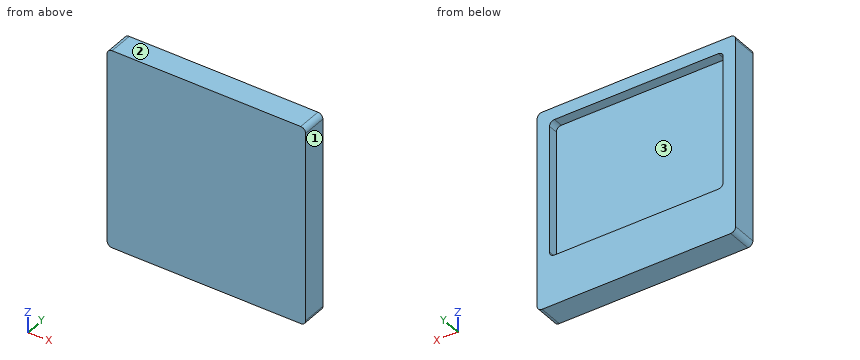
Autodesk Inventor part; units mm, degrees
ref_plane "YZ Plane" through (0, 0, 0) normal (1, 0, 0) x (0, 1, 0)
ref_plane "XZ Plane" through (0, 0, 0) normal (0, 1, 0) x (-1, 0, 0)
ref_plane "XY Plane" through (0, 0, 0) normal (0, 0, 1) x (1, 0, 0)
sketch "Sketch1" plane through (0, 0, 0) normal (0, 1, 0) x (-1, 0, 0)
  line L0 (0, 0) -> (80, 0)
  line L1 (80, 0) -> (80, -80)
  line L2 (80, -80) -> (0, -80)
  line L3 (0, -80) -> (0, 0)
  dimension "d0" = 80
  dimension "d1" = 80
extrude "Extrusion1" add sketch "Sketch1" along normal blind 6
sketch "Sketch2" plane through (0, 6, 0) normal (0, 1, 0) x (1, 0, 0)
  line L0 (-5, 5) -> (-75, 5)
  line L1 (-75, 5) -> (-75, 60)
  line L2 (-75, 60) -> (-5, 60)
  line L3 (-5, 60) -> (-5, 5)
  line L4 (0, 0) -> (0, 80)
  line L5 (-80, 0) -> (0, 0)
  line L6 (-80, 80) -> (-80, 0)
  line L7 (0, 80) -> (-80, 80)
  line L8 (-80, 0) -> (0, 0)
  line L9 (0, 0) -> (0, 80)
  line L10 (0, 80) -> (-80, 80)
  line L11 (-80, 80) -> (-80, 0)
  dimension "d8" = 70
  dimension "d9" = 55
  dimension "d10" = 5
  dimension "d11" = 5
extrude "Extrusion2" add sketch "Sketch2" along normal blind 4
fillet "Fillet1" radius 2 4 edges at (-75, 8, -60) (-5, 8, -60) (-5, 8, -5) (-75, 8, -5)
fillet "Fillet2" radius 2 4 edges at (0, 5, 0) (0, 5, -80) (-80, 5, -80) (-80, 5, 0)
properties part number "solar-panel-mount"
Source: CAD feature listing. Evaluate the final solid. Frame: model axes, mm. Face numbers are marked on the shaded views. Give positions to 0.01 mm unless a question says otherwise; leave off trailing zeros. Loops run counter-clockwise (first coordinate to the right, second up) from the corner with the lowest first, then second, coordinate; pieces in that order, holes last. Notation, with made-up numbers: M -22.75,83.25 L -13.75,83.25 A18 ccw -13.75,88.25 Z; hole C 87,37 d7. An arc over 180 degrees is marked long. Put each result on its own line as item: value.
Q1. Pin query (flat end, axial travel): P1, Ø4.5, axis at y = 7, z = -42.5, coming from the +X side. Return the tip coordinate at first contact, or that it passes through.
Response values:
P1: stops at x = 0
Q2. Section C-C (z = -10.5). Return the cut outline in (x, y), and give its area (3 significant figures).
Response values:
outline: M -80,0 L 0,0 L 0,10 L -5,10 L -5,6 L -75,6 L -75,10 L -80,10 Z
area: 520 mm²
Q3. Line query: probe 1 along X at (y, z) = (8, -54.5); probe 2 along Z at (x, y) = (-22, 8.75); probe 3 along Y at (x, z) = (-12, -8.5). Output: solid intervals per line, ascending. Write a range as [from, to].
Response values:
probe 1: x = [-80, -75], [-5, 0]
probe 2: z = [-80, -60], [-5, 0]
probe 3: y = [0, 6]
Q4. Section B-B (x = -16). Return the cut outline in (y, z), and give its area (3 significant figures).
Response values:
outline: M 0,-80 L 10,-80 L 10,-60 L 6,-60 L 6,-5 L 10,-5 L 10,0 L 0,0 Z
area: 580 mm²
Q5. Section A-A (y = 7.5). Return the cut outline in (x, z), and give its area (3 significant figures).
Response values:
outline: M -80,-78 A2 ccw -78,-80 L -2,-80 A2 ccw 0,-78 L 0,-2 A2 ccw -2,0 L -78,0 A2 ccw -80,-2 Z; hole M -75,-58 A2 ccw -73,-60 L -7,-60 A2 ccw -5,-58 L -5,-7 A2 ccw -7,-5 L -73,-5 A2 ccw -75,-7 Z
area: 2,550 mm²
Q6. Mould query, pull axis X, two halves, no side actions, for the marked faces 1, 2 and 3. Classes: released by +X, released by -X, zero draft, split by the parting line, or undercut.
Response values:
face 1: released by +X
face 2: zero draft
face 3: undercut
